from build123d import *

# Parameters (mm, degrees)
SKETCH1_R           = 50
SKETCH1_R_2         = 47.5
BOSS_EXTRUDE1_DEPTH = 20
SKETCH1_3_R         = 47.5
BOSS_EXTRUDE2_DEPTH = 4
SKETCH1_4_R         = 40
SKETCH1_4_R_2       = 16
SKETCH1_4_R_3       = 13.5
BOSS_EXTRUDE3_DEPTH = 15
SKETCH2_R           = 2
SKETCH2_R_2         = 1.5
CUT_EXTRUDE1_DEPTH  = 16


with BuildPart() as part:
    # Sketch1 → Boss-Extrude1 (new body)
    with BuildSketch(Plane(origin=(0, 0, 0), x_dir=(0, 0, -1), z_dir=(1, 0, 0))):
        Circle(SKETCH1_R)
        Circle(SKETCH1_R_2, mode=Mode.SUBTRACT)
    extrude(amount=BOSS_EXTRUDE1_DEPTH)

    # Sketch1_3 → Boss-Extrude2 (add)
    with BuildSketch(Plane(origin=(0, 0, 0), x_dir=(0, 0, -1), z_dir=(1, 0, 0))):
        Circle(SKETCH1_3_R)
        with BuildLine():
            ThreePointArc((15.714285714, 25.5550626), (17.117237545, 22.608325942), (15, 20.124611797))
            ThreePointArc((15, 20.124611797), (7.83467626, 16.36075337), (2.625, 10.166581284))
            ThreePointArc((2.625, 10.166581284), (0, 8.618950039), (-2.625, 10.166581284))
            ThreePointArc((-2.625, 10.166581284), (-7.83467626, 16.36075337), (-15, 20.124611797))
            ThreePointArc((-15, 20.124611797), (-17.117237545, 22.608325942), (-15.714285714, 25.5550626))
            ThreePointArc((-15.714285714, 25.5550626), (0, 30), (15.714285714, 25.5550626))
        make_face(mode=Mode.SUBTRACT)
        with BuildLine():
            ThreePointArc((-15.714285714, -25.5550626), (-17.117237545, -22.608325942), (-15, -20.124611797))
            ThreePointArc((-15, -20.124611797), (-7.83467626, -16.36075337), (-2.625, -10.166581284))
            ThreePointArc((-2.625, -10.166581284), (0, -8.618950039), (2.625, -10.166581284))
            ThreePointArc((2.625, -10.166581284), (7.83467626, -16.36075337), (15, -20.124611797))
            ThreePointArc((15, -20.124611797), (17.117237545, -22.608325942), (15.714285714, -25.5550626))
            ThreePointArc((15.714285714, -25.5550626), (0, -30), (-15.714285714, -25.5550626))
        make_face(mode=Mode.SUBTRACT)
    extrude(amount=BOSS_EXTRUDE2_DEPTH)

    # Sketch1_4 → Boss-Extrude3 (add)
    with BuildSketch(Plane(origin=(0, 0, 0), x_dir=(0, 0, -1), z_dir=(1, 0, 0))):
        Circle(SKETCH1_4_R)
        with Locations((-21, 0)):
            Circle(SKETCH1_4_R_2, mode=Mode.SUBTRACT)
        with Locations((21, 0)):
            Circle(SKETCH1_4_R_2, mode=Mode.SUBTRACT)
        with BuildLine():
            ThreePointArc((-15, -20.124611797), (-7.83467626, -16.36075337), (-2.625, -10.166581284))
            ThreePointArc((-2.625, -10.166581284), (0, -8.618950039), (2.625, -10.166581284))
            ThreePointArc((2.625, -10.166581284), (7.83467626, -16.36075337), (15, -20.124611797))
            ThreePointArc((15, -20.124611797), (17.117237545, -22.608325942), (15.714285714, -25.5550626))
            ThreePointArc((15.714285714, -25.5550626), (0, -30), (-15.714285714, -25.5550626))
            ThreePointArc((-15.714285714, -25.5550626), (-17.117237545, -22.608325942), (-15, -20.124611797))
        make_face(mode=Mode.SUBTRACT)
        with BuildLine():
            ThreePointArc((15.714285714, 25.5550626), (0, 30), (-15.714285714, 25.5550626))
            ThreePointArc((-15.714285714, 25.5550626), (-17.117237545, 22.608325942), (-15, 20.124611797))
            ThreePointArc((-15, 20.124611797), (-7.83467626, 16.36075337), (-2.625, 10.166581284))
            ThreePointArc((-2.625, 10.166581284), (0, 8.618950039), (2.625, 10.166581284))
            ThreePointArc((2.625, 10.166581284), (7.83467626, 16.36075337), (15, 20.124611797))
            ThreePointArc((15, 20.124611797), (17.117237545, 22.608325942), (15.714285714, 25.5550626))
        make_face(mode=Mode.SUBTRACT)
        with Locations((-21, 0)):
            Circle(SKETCH1_4_R_3)
        with Locations((21, 0)):
            Circle(SKETCH1_4_R_3)
    extrude(amount=BOSS_EXTRUDE3_DEPTH)

    # Sketch2 → Cut-Extrude1 (cut, through all)
    with BuildSketch(Plane(origin=(15, 0, 0), x_dir=(0, 0, -1), z_dir=(1, 0, 0))):
        with Locations((-27, -20)):
            Circle(SKETCH2_R)
        with Locations((-19, -28)):
            Circle(SKETCH2_R)
        with Locations((-20.508, 0)):
            Circle(SKETCH2_R_2)
        with Locations((-10.508, 0)):
            Circle(SKETCH2_R_2)
        with Locations((10, 0)):
            Circle(SKETCH2_R_2)
        with Locations((20, 0)):
            Circle(SKETCH2_R_2)
        with Locations((19, -28)):
            Circle(SKETCH2_R)
        with Locations((27, -20)):
            Circle(SKETCH2_R)
        with Locations((27, 20)):
            Circle(SKETCH2_R)
        with Locations((19, 28)):
            Circle(SKETCH2_R)
        with Locations((-19, 28)):
            Circle(SKETCH2_R)
        with Locations((-27, 20)):
            Circle(SKETCH2_R)
    extrude(amount=-CUT_EXTRUDE1_DEPTH, mode=Mode.SUBTRACT)


solid = part.part
Design review of the part built by this model. Coordinates are the model's own, in mm. A direction names the side the tool comes from. Give positions to 0.01 mm unless a question says otherwise; leave off trailing zeros. Loops run counter-clockwise (first coordinate to the right, second up) from the corner with the lowest first, then second, coordinate; pieces in that order, holes last. Notation, with made-up numbers: (-5.75, 53.5) - (11.25, 53.5) arc R28 cw to (11.25, 91.5) - close; hole circle Ø2 at (-33.5, -24). An arc over 180 degrees is marked (long way). Write item = value, one per line.
1) To check wall thickness, follow line 1 (Y direction, x = 7.25, z = 32); line 2 (Y direction, x = 3.25, z = -27); line 3 (Y direction, x = 12.5, z = 23). State the ranges of each line that lie inside material, in increasing order.
Result sheet:
line_1 = -38.42 to -35.1, -24 to -11.62, -7.83 to 7.83, 11.62 to 24, 35.1 to 38.42
line_2 = -42.08 to -22, -18 to 18, 22 to 42.08
line_3 = -44.4 to -41.56, -32.73 to -15.87, -13.35 to 13.35, 15.87 to 32.73, 41.56 to 44.4
2) Tool access review of faces 1 (the face through (7.4, -8.62, 0.04)), 2 (the face through (9.42, -39.05, 8.67)): name each direction out of +Z, -Z, +X, -X, +Y, -Y from which nothing blocks a thin tool from reaching the whole face with its end or side.
Result sheet:
face_1 = +X, -X
face_2 = +X
3) Take a section at A-A on z = 0. State the section outline as (x, y) points, and give its area (3 significant figures).
Result sheet:
outline = (0, -50) - (20, -50) - (20, -47.5) - (4, -47.5) - (4, -40) - (15, -40) - (15, -30) - (0, -30) - close; (0, -8.62) - (15, -8.62) - (15, 8.62) - (0, 8.62) - close; (0, 30) - (15, 30) - (15, 40) - (4, 40) - (4, 47.5) - (20, 47.5) - (20, 50) - (0, 50) - close
area = 719 mm2
4) Take a section at B-B on x = 5.5. Count the separate pieces of the cut face and the enclosed holes in it, and give its area (3 significant figures).
Result sheet:
separate_pieces = 4
enclosed_holes = 17
area = 4,350 mm2
5) Clearance check with flat-ended pins moving along their axes: pin 1 Ø10 at (x, z) = (15.5, -3.5) entering from -Y; pin 2 Ø3 at (x, y) = (12, 13) entering from +Z; pin 3 Ø2.5 at (y, z) = (0, 20.508) entering from -X; pin 4 Ø8 at (x, y) = (3.5, 9) entering from +Z. State where each tip first meets the part, or that it passes through.
Result sheet:
pin_1 = -50
pin_2 = 48.66
pin_3 = through
pin_4 = 49.75
6) Draft analysis for pull direction Z (two halves, no side actions). For faces 3 (the face through (7.395, -22.656, 17.123)), 4 (the face through (9.86, 15.02, -47.69)), 5 (the face through (8, 26, -19)), state which applies: +Z half, -Z half, draft (parallel to the pull), parting line (faces both ways), or undercut.
Result sheet:
face_3 = undercut
face_4 = parting line
face_5 = undercut
